The model under review builds one solid part; all positions refer to its coordinate system, in mm. A direction names the side the tool comes from. Give positions to 0.01 mm unless a question says otherwise; leave off trailing zeros. Order: outer loops, then holes, each group sorted by start corner. A loop starts at its lowest first (then second) coordinate and runs counter-clockwise, first axis right, second up. Notation, with made-up numbers: (-32.75, -34.5) - (20.25, -34.5) arc R24 cw to (20.25, 2.5) - close; hole circle Ø5 at (13, -15). An arc over 180 degrees is marked (long way). Put each result on its own line as item: value.
```python
from build123d import *

# Parameters (mm, degrees)
ESQUISSE1_W                                        = 150
ESQUISSE1_H                                        = 150
BOSS_EXTRU_1_DEPTH                                 = 25
CHAMBRAGE_POUR_VIS_T_TE_HEXAGONALE_M81_D           = 9
CHAMBRAGE_POUR_VIS_T_TE_HEXAGONALE_M81_CBORE_D     = 15
CHAMBRAGE_POUR_VIS_T_TE_HEXAGONALE_M81_CBORE_DEPTH = 8.6
CHAMBRAGE_POUR_VIS_T_TE_HEXAGONALE_M51_D           = 5.5
CHAMBRAGE_POUR_VIS_T_TE_HEXAGONALE_M51_CBORE_D     = 10
CHAMBRAGE_POUR_VIS_T_TE_HEXAGONALE_M51_CBORE_DEPTH = 5.4
ESQUISSE13_R                                       = 18.5
ENL_V_MAT_EXTRU_1_DEPTH                            = 22
ESQUISSE14_R                                       = 17
ENL_V_MAT_EXTRU_2_DEPTH                            = 4
ESQUISSE31_R                                       = 33
ENL_V_MAT_EXTRU_11_DEPTH                           = 5
TROU_POUR_TARAUDAGE_POUR_TROU_TARAUD_M6_D          = 5
TROU_POUR_TARAUDAGE_POUR_TROU_TARAUD_M6_DEPTH      = 16
TROU_POUR_TARAUDAGE_POUR_TROU_TARAUD_M6_TIP        = 1.502151548
ESQUISSE27_R                                       = 11
ENL_V_MAT_EXTRU_7_DEPTH                            = 18
ESQUISSE28_R                                       = 6.25
ENL_V_MAT_EXTRU_8_DEPTH                            = 8
ENL_V_MAT_EXTRU_9_DEPTH                            = 20.6
ENL_V_MAT_EXTRU_10_DEPTH                           = 5.4
ESQUISSE32_R                                       = 129.983308099
ESQUISSE32_W                                       = 140
ESQUISSE32_H                                       = 140
ENL_V_MAT_EXTRU_12_DEPTH                           = 26


with BuildPart() as part:
    # Esquisse1 → Boss.-Extru.1 (new body)
    with BuildSketch(Plane.XY):
        Rectangle(ESQUISSE1_W, ESQUISSE1_H)
    extrude(amount=BOSS_EXTRU_1_DEPTH)

    # Chambrage pour vis à tête hexagonale M81 (through all)
    with Locations(Plane(origin=(0, 0, 0), x_dir=(-1, 0, 0), z_dir=(0, 0, -1))):
        with Locations((-57.5, -57.5), (-57.5, 57.5)):
            CounterBoreHole(CHAMBRAGE_POUR_VIS_T_TE_HEXAGONALE_M81_D / 2, CHAMBRAGE_POUR_VIS_T_TE_HEXAGONALE_M81_CBORE_D / 2, CHAMBRAGE_POUR_VIS_T_TE_HEXAGONALE_M81_CBORE_DEPTH)

    # Chambrage pour vis à tête hexagonale M51 (through all)
    with Locations(Plane(origin=(0, 0, 0), x_dir=(-1, 0, 0), z_dir=(0, 0, -1))):
        with Locations((14.144188312, -59.37), (61.284188312, -59.37), (61.284188312, -12.23)):
            CounterBoreHole(CHAMBRAGE_POUR_VIS_T_TE_HEXAGONALE_M51_D / 2, CHAMBRAGE_POUR_VIS_T_TE_HEXAGONALE_M51_CBORE_D / 2, CHAMBRAGE_POUR_VIS_T_TE_HEXAGONALE_M51_CBORE_DEPTH)

    # Esquisse13 → Enlèv. mat.-Extru.1 (cut)
    with BuildSketch(Plane.XY):
        Circle(ESQUISSE13_R)
    extrude(amount=ENL_V_MAT_EXTRU_1_DEPTH, mode=Mode.SUBTRACT)

    # Esquisse14 → Enlèv. mat.-Extru.2 (cut, through all)
    with BuildSketch(Plane(origin=(0, 0, 22), x_dir=(-1, 0, 0), z_dir=(0, 0, -1))):
        Circle(ESQUISSE14_R)
    extrude(amount=-ENL_V_MAT_EXTRU_2_DEPTH, mode=Mode.SUBTRACT)

    # Esquisse31 → Enlèv. mat.-Extru.11 (cut)
    with BuildSketch(Plane(origin=(0, 0, 0), x_dir=(-1, 0, 0), z_dir=(0, 0, -1))):
        Circle(ESQUISSE31_R)
    extrude(amount=-ENL_V_MAT_EXTRU_11_DEPTH, mode=Mode.SUBTRACT)

    # Trou pour taraudage pour trou taraudé M61
    with Locations(Plane(origin=(0, 0, 5), x_dir=(1, 0, 0), z_dir=(0, 0, -1))):
        with Locations((0, 25), (-25, 0), (0, -25), (25, 0), (0, 0)):
            Hole(TROU_POUR_TARAUDAGE_POUR_TROU_TARAUD_M6_D / 2, depth=TROU_POUR_TARAUDAGE_POUR_TROU_TARAUD_M6_DEPTH)
            with Locations((0, 0, -(TROU_POUR_TARAUDAGE_POUR_TROU_TARAUD_M6_DEPTH + TROU_POUR_TARAUDAGE_POUR_TROU_TARAUD_M6_TIP / 2))):  # 118° drill point
                Cone(0, TROU_POUR_TARAUDAGE_POUR_TROU_TARAUD_M6_D / 2, TROU_POUR_TARAUDAGE_POUR_TROU_TARAUD_M6_TIP, mode=Mode.SUBTRACT)

    # Esquisse27 → Enlèv. mat.-Extru.7 (cut)
    with BuildSketch(Plane(origin=(0, 0, 0), x_dir=(-1, 0, 0), z_dir=(0, 0, -1))):
        with Locations((-30, -43.084219849)):
            Circle(ESQUISSE27_R)
    extrude(amount=-ENL_V_MAT_EXTRU_7_DEPTH, mode=Mode.SUBTRACT)

    # Esquisse28 → Enlèv. mat.-Extru.8 (cut, through all)
    with BuildSketch(Plane(origin=(0, 0, 18), x_dir=(-1, 0, 0), z_dir=(0, 0, -1))):
        with Locations((-30, -43.084219849)):
            Circle(ESQUISSE28_R)
    extrude(amount=-ENL_V_MAT_EXTRU_8_DEPTH, mode=Mode.SUBTRACT)

    # Esquisse29 → Enlèv. mat.-Extru.9 (cut, through all)
    with BuildSketch(Plane(origin=(0, 0, 5.4), x_dir=(-1, 0, 0), z_dir=(0, 0, -1))):
        with BuildLine():
            Line((61.284188312, -62.12), (43.284188312, -62.12))
            ThreePointArc((43.284188312, -62.12), (40.534188312, -59.37), (43.284188312, -56.62))
            Line((43.284188312, -56.62), (61.284188312, -56.62))
            ThreePointArc((61.284188312, -56.62), (64.034188312, -59.37), (61.284188312, -62.12))
        make_face()
        with BuildLine():
            Line((14.144188312, -62.12), (-3.855811688, -62.12))
            ThreePointArc((-3.855811688, -62.12), (-6.605811688, -59.37), (-3.855811688, -56.62))
            Line((-3.855811688, -56.62), (14.144188312, -56.62))
            ThreePointArc((14.144188312, -56.62), (16.894188312, -59.37), (14.144188312, -62.12))
        make_face()
        with BuildLine():
            Line((61.284188312, -14.98), (43.284188312, -14.98))
            ThreePointArc((43.284188312, -14.98), (40.534188312, -12.23), (43.284188312, -9.48))
            Line((43.284188312, -9.48), (61.284188312, -9.48))
            ThreePointArc((61.284188312, -9.48), (64.034188312, -12.23), (61.284188312, -14.98))
        make_face()
    extrude(amount=-ENL_V_MAT_EXTRU_9_DEPTH, mode=Mode.SUBTRACT)

    # Esquisse30 → Enlèv. mat.-Extru.10 (cut)
    with BuildSketch(Plane(origin=(0, 0, 0), x_dir=(-1, 0, 0), z_dir=(0, 0, -1))):
        with BuildLine():
            Line((-3.855811688, -64.37), (14.144188312, -64.37))
            ThreePointArc((14.144188312, -64.37), (19.144188312, -59.37), (14.144188312, -54.37))
            Line((14.144188312, -54.37), (-3.855811688, -54.37))
            ThreePointArc((-3.855811688, -54.37), (-8.855811688, -59.37), (-3.855811688, -64.37))
        make_face()
        with BuildLine():
            Line((43.284188312, -64.37), (61.284188312, -64.37))
            ThreePointArc((61.284188312, -64.37), (66.284188312, -59.37), (61.284188312, -54.37))
            Line((61.284188312, -54.37), (43.284188312, -54.37))
            ThreePointArc((43.284188312, -54.37), (38.284188312, -59.37), (43.284188312, -64.37))
        make_face()
        with BuildLine():
            Line((43.284188312, -17.23), (61.284188312, -17.23))
            ThreePointArc((61.284188312, -17.23), (66.284188312, -12.23), (61.284188312, -7.23))
            Line((61.284188312, -7.23), (43.284188312, -7.23))
            ThreePointArc((43.284188312, -7.23), (38.284188312, -12.23), (43.284188312, -17.23))
        make_face()
    extrude(amount=-ENL_V_MAT_EXTRU_10_DEPTH, mode=Mode.SUBTRACT)

    # Esquisse32 → Enlèv. mat.-Extru.12 (cut, through all)
    with BuildSketch(Plane(origin=(0, 0, 0), x_dir=(-1, 0, 0), z_dir=(0, 0, -1))):
        Circle(ESQUISSE32_R)
        Rectangle(ESQUISSE32_W, ESQUISSE32_H, mode=Mode.SUBTRACT)
    extrude(amount=-ENL_V_MAT_EXTRU_12_DEPTH, mode=Mode.SUBTRACT)


solid = part.part
```
(1) Take a section at C-C, the plane z = 12.25. Count the separate pieces of the cut face and the enclosed holes in it, then the cut area to 3 significant figures.
The answers:
separate pieces: 1
enclosed holes: 11
area: 17,600 mm^2
(2) Take a section at B-B, the plane y = -12.23. Write out the cut boundary in (x, z).
The answers:
outline: (-70, 0) - (-66.28, 0) - (-66.28, 5.4) - (-64.03, 5.4) - (-64.03, 25) - (-70, 25) - close; (-40.53, 5.4) - (-38.28, 5.4) - (-38.28, 0) - (-30.65, 0) - (-30.65, 5) - (-13.88, 5) - (-13.88, 22) - (-11.81, 22) - (-11.81, 25) - (-40.53, 25) - close; (11.81, 22) - (13.88, 22) - (13.88, 5) - (30.65, 5) - (30.65, 0) - (70, 0) - (70, 25) - (11.81, 25) - close
(3) The part is to be moulded in two halves that separate along X. For faces 1 (the cylindrical face through (24.1, -33.8, 8.9)), 2 (the flat face through (70, -1, 12)), 3 (the flat face through (1, 70, 12)), say which applies: pulls with the +X half, pulls with the -X half, needs draft (parallel to the pull), parting line crosses it, or undercut.
The answers:
face 1: undercut
face 2: pulls with the +X half
face 3: needs draft
(4) Clearance check with flat-ended pins moving along their axes: pin 1 Ø20 at (x, y) = (-5, 3.5) entering from -Z; pin 2 Ø13 at (x, y) = (30, -43.08) entering from -Z; pin 3 Ø7.5 at (x, y) = (58, 55) entering from -Z; pin 4 Ø5 at (x, y) = (-48, -60.5) entering from -Z. State where each tip first meets the part, or that it passes through.
The answers:
pin 1: through
pin 2: z = 18
pin 3: z = 8.6
pin 4: z = 5.4
(5) Take a section at A-A, the plane x = 57.5. Write out the cut boundary in (y, z), then the cut area to 3 significant figures.
The answers:
outline: (-70, 0) - (-65, 0) - (-65, 8.6) - (-62, 8.6) - (-62, 25) - (-70, 25) - close; (-53, 8.6) - (-50, 8.6) - (-50, 0) - (50, 0) - (50, 8.6) - (53, 8.6) - (53, 25) - (-53, 25) - close; (62, 8.6) - (65, 8.6) - (65, 0) - (70, 0) - (70, 25) - (62, 25) - close
area: 2,950 mm^2
(6) For faces 4 (the flat face through (15, 17, 25)), 5 (the cylindrical face through (58.476, 64.936, 4.24)), 6 (the cylindrical face through (6.605, -59.43, 15.063)), list the 3-axis set-ups (+Z, -Z, +X, -X, +Y, -Y) from which the entire face can be reached by the end or side of a thin tool; tool diameter is ignored.
The answers:
face 4: +Z, +X, -X, +Y, -Y
face 5: -Z
face 6: +Z, -Z
(7) Wall thickness on L1, parallel to Y at x = 57.5, z = 14.75; L2, parallel to Y at x = 0, z = 23.05; L3, parallel to Z at x = 39, y = -39.5: over which ranges is each line inside the solid? List them lowest first.
The answers:
L1: -70 to -62, -53 to 53, 62 to 70
L2: -70 to -62.12, -56.62 to -17, 17 to 70
L3: 18 to 25
